from build123d import *

# Parameters (mm, degrees)
F0_W      = 63.5
F0_H      = 63.5
F1_DEPTH  = 6.35
F2_W      = 54.863996
F2_H      = 52.120802
F3_DEPTH  = 5.08
F4_W      = 45.72
F4_H      = 41.148004
F5_DEPTH  = 5.08
F6_W      = 35.356802
F6_H      = 32.613602
F7_DEPTH  = 5.08
F8_W      = 24.461082
F8_H      = 22.671008
F9_DEPTH  = 5.08
F10_W     = 18.8976
F10_H     = 14.9352
F11_DEPTH = 25.4
F12_W     = 4.960672
F12_H     = 7.49556
F13_DEPTH = 39.37
F14_W     = 2.972535
F14_H     = 6.727309
F15_DEPTH = 2.54


with BuildPart() as f1:
    # F0 (on Top) → F1 (new body)
    with BuildSketch(Plane.XY):
        Rectangle(F0_W, F0_H)
    extrude(amount=F1_DEPTH)

    # F2 (on face) → F3 (join)
    with BuildSketch(Plane.XY.offset(6.35)):
        Rectangle(F2_W, F2_H)
    extrude(amount=F3_DEPTH)

    # F4 (on face) → F5 (join)
    with BuildSketch(Plane.XY.offset(11.43)):
        Rectangle(F4_W, F4_H)
    extrude(amount=F5_DEPTH)

    # F6 (on face) → F7 (join)
    with BuildSketch(Plane.XY.offset(16.51)):
        Rectangle(F6_W, F6_H)
    extrude(amount=F7_DEPTH)

    # F8 (on face) → F9 (join)
    with BuildSketch(Plane.XY.offset(21.59)):
        Rectangle(F8_W, F8_H)
    extrude(amount=F9_DEPTH)

    # F10 (on face) → F11 (join)
    with BuildSketch(Plane.XY.offset(26.67)):
        Rectangle(F10_W, F10_H)
    extrude(amount=F11_DEPTH)

    # F12 (on face) → F13 (cut)
    with BuildSketch(Plane.XZ.offset(7.4676)):
        with Locations((0, 42.749591)):
            Rectangle(F12_W, F12_H)
    extrude(amount=-F13_DEPTH, mode=Mode.SUBTRACT)

    # F14 (on face) → F15 (cut)
    with BuildSketch(Plane(origin=(-9.4488, 0, 0), x_dir=(0, -1, 0), z_dir=(-1, 0, 0))):
        with Locations((-0.047928, 30.033654)):
            Rectangle(F14_W, F14_H)
    extrude(amount=-F15_DEPTH, mode=Mode.SUBTRACT)


solid = f1.part
The listing builds one solid part. Answer for the finished solid, in the listing's coordinates (mm). A direction names the side the tool comes from. Give positions to 0.01 mm unless a question says otherwise; leave off trailing zeros. Loops run counter-clockwise (first coordinate to the right, second up) from the corner with the lowest first, then second, coordinate; pieces in that order, holes last. Notation, with made-up numbers: M 88,4 L 109,4 A36 ccw 109,41 Z; hole C -12,53.25 d6. An arc over 180 degrees is marked long. Answer as CSV lines item,"result".
Item 1: Straight lines are drawn through the part: line 1 along Y through (x, z) = (15, 17); line 2 along X through (y, z) = (-1.5, 27); line 3 along X through (y, z) = (19, 10). For each, find the intervals that lie inside material, in ascending order. Write a range as [from, to].
Values follow:
line 1,"y = [-16.31, 16.31]"
line 2,"x = [-9.45, 9.45]"
line 3,"x = [-27.43, 27.43]"
Item 2: The part is cut by section B-B (z = 29). Give the vertices of the cut face in (x, y), and give its area (3 significant figures).
Values follow:
outline,"M -9.45,-7.47 L 9.45,-7.47 L 9.45,7.47 L -9.45,7.47 L -9.45,1.53 L -6.91,1.53 L -6.91,-1.44 L -9.45,-1.44 Z"
area,"275 mm^2"
Item 3: The part is cut by section C-C (y = -12.5). Give the vertices of the cut face in (x, z), and give its area (3 significant figures).
Values follow:
outline,"M -31.75,0 L 31.75,0 L 31.75,6.35 L 27.43,6.35 L 27.43,11.43 L 22.86,11.43 L 22.86,16.51 L 17.68,16.51 L 17.68,21.59 L -17.68,21.59 L -17.68,16.51 L -22.86,16.51 L -22.86,11.43 L -27.43,11.43 L -27.43,6.35 L -31.75,6.35 Z"
area,"1,090 mm^2"
Item 4: The part is cut by section D-D (x = 26.5). Give the vertices of the cut face in (y, z).
Values follow:
outline,"M -31.75,0 L 31.75,0 L 31.75,6.35 L 26.06,6.35 L 26.06,11.43 L -26.06,11.43 L -26.06,6.35 L -31.75,6.35 Z"
Item 5: The mould has two halves that part along X. Classify faces 4 (the flat face through (-22.86, 0, 14)), 5 (the flat face through (0, -14, 21.59)), 6 (the flat face through (0, 0, 46.497)): released by +X, released by -X, zero draft, split by the parting line, or undercut.
Values follow:
face 4,"released by -X"
face 5,"zero draft"
face 6,"undercut"
Item 6: Given pin 1 Ø2.5 at (x, z) = (8.5, 18) entering from +Y; pin 2 Ø5.5 at (x, z) = (0.5, 23.5) entering from -Y; pin 3 Ø3 at (x, y) = (11.5, 7) entering from -Z; pin 4 Ø2.5 at (x, z) = (-1, 14) entering from -Y, each flat-ended and moving along its own axis, determine where each tip first touches the part or whether it passes through.
Values follow:
pin 1,"stops at y = 16.31"
pin 2,"stops at y = -16.31"
pin 3,"stops at z = 0"
pin 4,"stops at y = -20.57"
Item 7: Which of the six approach directions +Z, -Z, +X, -X, +Y, -Y give full straight-line access (tool end or side, diameter ignored) to faces 1 (the flat face through (0, -11.336, 24)), 2 (the flat face through (2.48, 0, 43)), 3 (the flat face through (-9.449, 0, 39))?
Values follow:
face 1,"+Z, +X, -X, -Y"
face 2,"+Y, -Y"
face 3,"+Z, -X, +Y, -Y"
Item 8: The part is cut by section A-A (x = 1.5). Give the vertices of the cut face in (y, z), and give its area (3 significant figures).
Values follow:
outline,"M -31.75,0 L 31.75,0 L 31.75,6.35 L 26.06,6.35 L 26.06,11.43 L 20.57,11.43 L 20.57,16.51 L 16.31,16.51 L 16.31,21.59 L 11.34,21.59 L 11.34,26.67 L 7.47,26.67 L 7.47,39 L -7.47,39 L -7.47,26.67 L -11.34,26.67 L -11.34,21.59 L -16.31,21.59 L -16.31,16.51 L -20.57,16.51 L -20.57,11.43 L -26.06,11.43 L -26.06,6.35 L -31.75,6.35 Z; M -7.47,46.5 L 7.47,46.5 L 7.47,52.07 L -7.47,52.07 Z"
area,"1,430 mm^2"
